Read the model definition and answer for the solid it produces. Units are mm, in the model's axes. Face numbers are marked on the shaded views. A direction names the side the tool comes from. Coordinates: 2 decimals unless noted, no trailing zeros. Order: outer loops, then holes, each group sorted by start corner. A loop starts at its lowest first (then second) coordinate and runs counter-clockwise, first axis right, second up. Notation, with made-up numbers: M -10,61 L 44,61 A5 ccw 44,70 Z; hole C -11.75,-10.5 d9. An arc over 180 degrees is marked long. Write each question's results on one line, items separated by ' | '.
```python
from build123d import *

# Parameters (mm, degrees)
SKETCH_1_R          = 19
EXTRUDE_1_DEPTH     = 34
SKETCH_2_R          = 10
EXTRUDE_2_DEPTH     = 5
SKETCH_3_R          = 4
EXTRUDE_3_DEPTH     = 1
SKETCH_4_R          = 3
EXTRUDE_4_DEPTH     = 15.5
CUT_EXTRUDE_2_DEPTH = 12
SKETCH_7_R          = 1.5
CUT_EXTRUDE_3_DEPTH = 6


with BuildPart() as part:
    # 草图1 → 凸台-拉伸1 (new body)
    with BuildSketch(Plane.XY):
        Circle(SKETCH_1_R)
    extrude(amount=EXTRUDE_1_DEPTH)

    # 草图2 → 凸台-拉伸2 (add)
    with BuildSketch(Plane(origin=(0, 0, 0), x_dir=(-1, 0, 0), z_dir=(0, 0, -1))):
        Circle(SKETCH_2_R)
    extrude(amount=EXTRUDE_2_DEPTH)

    # 草图3 → 凸台-拉伸3 (add)
    with BuildSketch(Plane(origin=(0, 0, -5), x_dir=(-1, 0, 0), z_dir=(0, 0, -1))):
        Circle(SKETCH_3_R)
    extrude(amount=EXTRUDE_3_DEPTH)

    # 草图4 → 凸台-拉伸4 (add)
    with BuildSketch(Plane(origin=(0, 0, -6), x_dir=(-1, 0, 0), z_dir=(0, 0, -1))):
        Circle(SKETCH_4_R)
    extrude(amount=EXTRUDE_4_DEPTH)

    # 草图5 → 切除-拉伸2 (cut)
    with BuildSketch(Plane(origin=(0, 0, -21.5), x_dir=(-1, 0, 0), z_dir=(0, 0, -1))):
        with BuildLine():
            ThreePointArc((1.658312395, 2.5), (0.866025404, 2.872281323), (0, 3))
            Line((0, 3), (0, 2.5))
            Line((0, 2.5), (1.658312395, 2.5))
        make_face()
        with BuildLine():
            Line((0, 2.5), (0, 3))
            ThreePointArc((0, 3), (-0.866025404, 2.872281323), (-1.658312395, 2.5))
            Line((-1.658312395, 2.5), (0, 2.5))
        make_face()
    extrude(amount=-CUT_EXTRUDE_2_DEPTH, mode=Mode.SUBTRACT)

    # 草图7 → 切除-拉伸3 (cut)
    with BuildSketch(Plane(origin=(0, 0, 0), x_dir=(-1, 0, 0), z_dir=(0, 0, -1))):
        with Locations((0, 15)):
            Circle(SKETCH_7_R)
        with Locations((-12.990381057, -7.5)):
            Circle(SKETCH_7_R)
        with Locations((12.990381057, -7.5)):
            Circle(SKETCH_7_R)
    extrude(amount=-CUT_EXTRUDE_3_DEPTH, mode=Mode.SUBTRACT)


solid = part.part
```
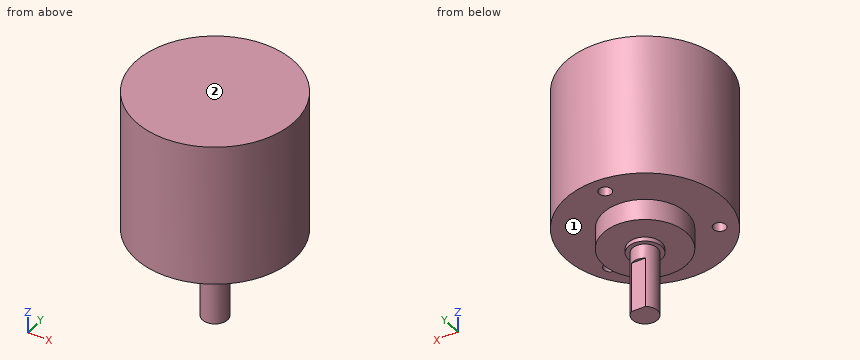
(1) The part is cut by section C-C, the plane z = -3.5. Write down the section's boundary in (x, y), then the cut area to 3 significant figures.
Conclusion:
outline: C 0,0 d20 | area: 314 mm²
(2) Given pin 1 (2.5 mm diameter, centred on x = 12.99, y = -7.5, fed in from -Z); pin 2 (2 mm diameter, centred on x = 12.5, z = -6.5, fed in from -Y); pin 3 (3.5 mm diameter, centred on x = -12.99, y = -7.5, fed in from -Z); pin 4 (5 mm diameter, centred on y = -9, z = 11, fed in from -X), each flat-ended and moving along its own axis, determine where each tip first touches the part or whether it passes through.
Conclusion:
pin 1: z = 6 | pin 2: through | pin 3: z = 0 | pin 4: x = -17.85
(3) The part is cut by section B-B, the plane y = 0. Write down the section's boundary in (x, z).
Conclusion:
outline: M -19,0 L -10,0 L -10,-5 L -4,-5 L -4,-6 L -3,-6 L -3,-21.5 L 3,-21.5 L 3,-6 L 4,-6 L 4,-5 L 10,-5 L 10,0 L 19,0 L 19,34 L -19,34 Z
(4) The part is cut by section D-D, the plane x = 6. Write down the section's boundary in (y, z).
Conclusion:
outline: M -18.03,0 L -8,0 L -8,-5 L 8,-5 L 8,0 L 18.03,0 L 18.03,34 L -18.03,34 Z
(5) The part is cut by section A-A, the plane x = 0. Write down the section's boundary in (y, z), then the cut area to 3 significant figures.
Conclusion:
outline: M -19,0 L -10,0 L -10,-5 L -4,-5 L -4,-6 L -3,-6 L -3,-21.5 L 2.5,-21.5 L 2.5,-9.5 L 3,-9.5 L 3,-6 L 4,-6 L 4,-5 L 10,-5 L 10,0 L 13.5,0 L 13.5,6 L 16.5,6 L 16.5,0 L 19,0 L 19,34 L -19,34 Z | area: 1,470 mm²
(6) For the marked faces 1 and 2, determine the directions among +Z, -Z, +X, -X, +Y, -Y from which every point of the face is accessible in a straight line to the end or side of a thin tool.
Conclusion:
face 1: -Z | face 2: +Z, +X, -X, +Y, -Y
(7) Straight lines are drawn through the part: line 1 (Z direction, x = -4, y = -2); line 2 (Y direction, x = 0.5, z = 7.5); line 3 (Z direction, x = 16, y = 2). For each, find the intervals that lie inside material, in ascending order.
Conclusion:
line 1: -5 to 34 | line 2: -18.99 to 18.99 | line 3: 0 to 34
